Verification items for this drawing (mm, ordinates from the low corner). Give positions to 0.01 mm unless a question says otherwise; leave off trailing zeros. Loops run counter-clockwise (first coordinate to the right, second up) from the corner with the lowest first, then second, coordinate; pieces in that order, holes last. Notation, with made-up numbers: (0, -15.5) -> (26, -15.5) arc R22 ccw to (26, 23.5) -> close; hole circle Ø1 at (-24, -22). An arc over 180 degrees is marked (long way). Write each question's results on one line, items separated by ' | '. Start each with the question number.
1) Scan lines: line 1 (X direction, y = 1.45, z = 25); line 2 (Z direction, x = 15, y = 1); line 3 (X direction, y = 1.5, z = 43.5). Record each from-to range of solid material in increasing order. Write a range as from..to.
2) Depth check by flat-ended pin: pin 1 (2.5 mm diameter, centred on x = 25, z = 25, fed in from -Y). Enter the tip coordinate at first touch or a pass-through.
3) Sectioned sample at A-A on x = 15. Record the cut outline in (y, z), then the cut area to 3 significant figures.
4) Sectioned sample at B-B on z = 25. Record the cut outline in (x, y).
5) Sectioned sample at C-C on y = 0.85. Record the cut outline in (x, z), then the cut area to 3 significant figures.
6) Sectioned sample at D-D on x = 26. Record the cut outline in (y, z), then the cut area to 3 significant figures.
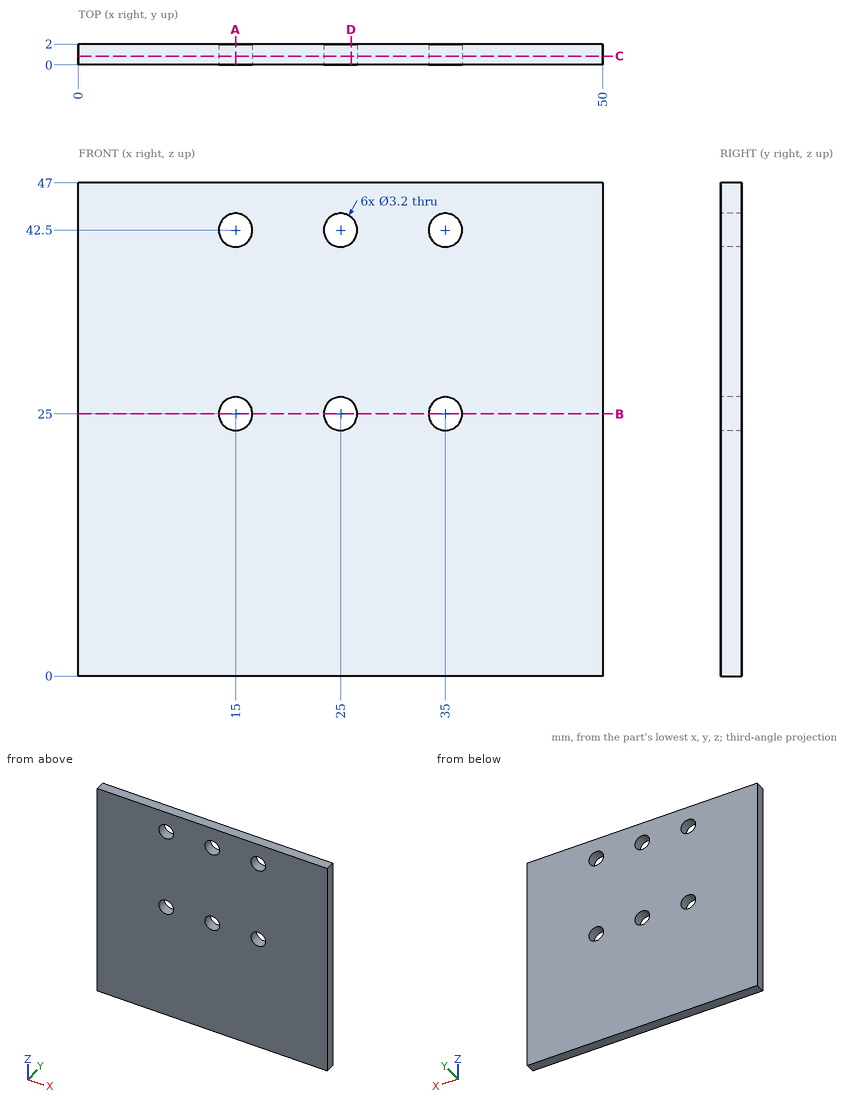
Result:
1) line 1: 0..13.4, 16.6..23.4, 26.6..33.4, 36.6..50 | line 2: 0..23.4, 26.6..40.9, 44.1..47 | line 3: 0..13.75, 16.25..23.75, 26.25..33.75, 36.25..50
2) pin 1: through
3) outline: (0, 0) -> (2, 0) -> (2, 23.4) -> (0, 23.4) -> close; (0, 26.6) -> (2, 26.6) -> (2, 40.9) -> (0, 40.9) -> close; (0, 44.1) -> (2, 44.1) -> (2, 47) -> (0, 47) -> close | area: 81.2 mm^2
4) outline: (0, 0) -> (13.4, 0) -> (13.4, 2) -> (0, 2) -> close; (16.6, 0) -> (23.4, 0) -> (23.4, 2) -> (16.6, 2) -> close; (26.6, 0) -> (33.4, 0) -> (33.4, 2) -> (26.6, 2) -> close; (36.6, 0) -> (50, 0) -> (50, 2) -> (36.6, 2) -> close
5) outline: (0, 0) -> (50, 0) -> (50, 47) -> (0, 47) -> close; hole circle Ø3.2 at (15, 25); hole circle Ø3.2 at (15, 42.5); hole circle Ø3.2 at (25, 25); hole circle Ø3.2 at (25, 42.5); hole circle Ø3.2 at (35, 25); hole circle Ø3.2 at (35, 42.5) | area: 2,300 mm^2
6) outline: (0, 0) -> (2, 0) -> (2, 23.75) -> (0, 23.75) -> close; (0, 26.25) -> (2, 26.25) -> (2, 41.25) -> (0, 41.25) -> close; (0, 43.75) -> (2, 43.75) -> (2, 47) -> (0, 47) -> close | area: 84.0 mm^2
